The drawing under review shows one solid part. Ordinate dimensions are in mm from its lowest x, y, z. Round coordinates to 2 decimals unless told otherwise and drop trailing zeros. Write each loop counter-clockwise with the first axis right and the second up, starting at its lowest first coordinate (ties: lowest second). Pieces come first, ordered by that corner, then holes. Notation, with made-up numbers: (50.25, -17.75) - (101.25, -17.75) arc R25 cw to (101.25, 0.25) - close; hole circle Ø8 at (-10, 28.25). An arc over 180 degrees is marked (long way). One line per question, with ' | ' between items. Start each with the question number.
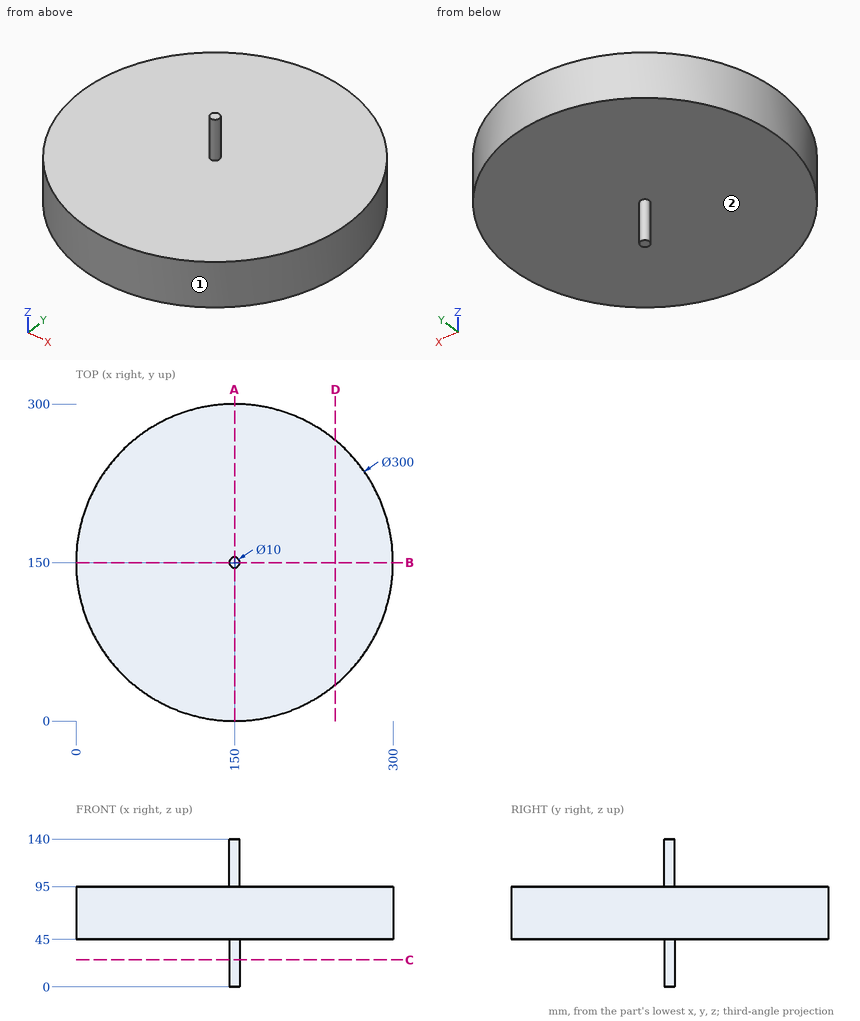
1. Add section C-C, the plane z = 25.5. Write out the cut boundary in (x, y), then the cut area to 3 significant figures.
2. The part is to be moulded in two halves that separate along Y. For the marked faces 1 and 2, say which applies: pulls with the +Y half, pulls with the -Y half, needs draft (parallel to the pull), parting line crosses it, or undercut.
3. Add section A-A, the plane x = 150. Write out the cut boundary in (y, z).
4. Add section D-D, the plane x = 245.5. Write out the cut boundary in (y, z), then the cut area to 3 significant figures.
5. Clearance check with flat-ended pins moving along their axes: P1, Ø8, axis at x = 258, y = 250, coming from the +Z side; P2, Ø8, axis at y = 217.5, z = 97.5, coming from the -X side; P3, Ø5, axis at x = 247, y = 201, coming from the -Z side. State where each tip first meets the part, or that it passes through.
6. Wall thickness on line 1 along Z through (x, y) = (137.5, 185.5); line 2 along Y through (x, z) = (153.5, 81.5); line 3 along Y through (x, z) = (242.5, 93): over which ranges is each line inside the solid? List them lowest first. Write a range as [from, to].
Geometry check:
1) outline: circle Ø10 at (150, 150) | area: 78.5 mm2
2) face 1: parting line crosses it | face 2: needs draft
3) outline: (0, 45) - (145, 45) - (145, 0) - (155, 0) - (155, 45) - (300, 45) - (300, 95) - (155, 95) - (155, 140) - (145, 140) - (145, 95) - (0, 95) - close
4) outline: (34.33, 45) - (265.67, 45) - (265.67, 95) - (34.33, 95) - close | area: 11,600 mm2
5) P1: stops at z = 95 | P2: stops at x = 14.52 | P3: stops at z = 45
6) line 1: z = [45, 95] | line 2: y = [0.04, 299.96] | line 3: y = [31.92, 268.08]
